Autodesk Inventor part; units mm, degrees
ref_plane "YZ Plane" through (0, 0, 0) normal (1, 0, 0) x (0, 1, 0)
ref_plane "XZ Plane" through (0, 0, 0) normal (0, 1, 0) x (-1, 0, 0)
ref_plane "XY Plane" through (0, 0, 0) normal (0, 0, 1) x (1, 0, 0)
sketch "Sketch1" plane through (0, 0, 0) normal (1, 0, 0) x (0, 1, 0)
  line L0 (0, 24.9554) -> (36.4449, 24.9554)
  arc A0 (31.5833, 1.489) -> (36.4449, 24.9554) centre (37.5, 12.5) ccw
  arc A1 (31.7956, 1.3803) -> (0, 9.582) centre (-2.2398, -64.8326) ccw
  circle A2 centre (37.5, 3.991) radius 1.25
  circle A3 centre (28.991, 12.5) radius 1.25
  circle A4 centre (37.5, 21.009) radius 1.25
  circle A5 centre (46.009, 12.5) radius 1.25
  circle A6 centre (28.6546, 17.1646) radius 1.25
  circle A7 centre (20.6937, 21.3627) radius 1.25
  circle A8 centre (37.5, 12.5) radius 4.5
  line L1 (-2.2398, 24.9554) -> (-2.25, 24.9554)
  arc A9 (-2.2398, 9.6157) -> (-2.25, 9.6157) centre (-2.2398, -64.8326) ccw
  arc A10 (0, 9.582) -> (-31.7956, 1.3803) centre (2.2398, -64.8326) ccw
  line L2 (0, 24.9554) -> (-36.4449, 24.9554)
  arc A11 (-36.4449, 24.9554) -> (-31.5833, 1.489) centre (-37.5, 12.5) ccw
  circle A12 centre (-37.5, 3.991) radius 1.25
  circle A13 centre (-28.991, 12.5) radius 1.25
  circle A14 centre (-37.5, 21.009) radius 1.25
  circle A15 centre (-46.009, 12.5) radius 1.25
  circle A16 centre (-28.6546, 17.1646) radius 1.25
  circle A17 centre (-20.6937, 21.3627) radius 1.25
  circle A18 centre (-37.5, 12.5) radius 4.5
  line L3 (2.2398, 24.9554) -> (2.25, 24.9554)
  arc A19 (2.25, 9.6157) -> (2.2398, 9.6157) centre (2.2398, -64.8326) ccw
  point P0 (0.0204, 0)
  point P1 (-0.0204, 0)
  dimension "d47" = 8.509
  dimension "d48" = 8.509
  dimension "d49" = 8.509
  dimension "d50" = 8.509
  dimension "d51" = 10
  dimension "d53" = 9
  dimension "d56" = 9
  dimension "d58" = 4.1981
  dimension "d61" = 75
extrude "Extrusion3" add sketch "Sketch1" along normal mid plane 3.5
properties part number "tibia extrude"
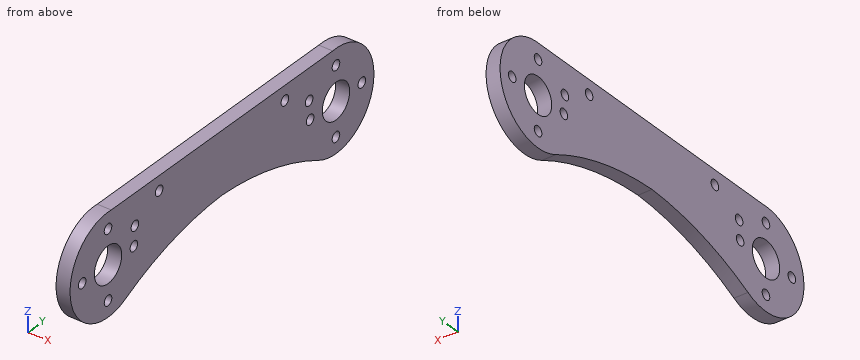
Work out the finished part from the listing and answer in its coordinate system (mm). Give positions to 0.01 mm unless a question says otherwise; leave off trailing zeros. Order: outer loops, then holes, each group sorted by start corner. A loop starts at its lowest first (then second) coordinate and runs counter-clockwise, first axis right, second up. Notation, with made-up numbers: (83.5, 87) -> (117.5, 87) arc R26 ccw to (117.5, 121) -> close; hole circle Ø6 at (55, 18). An arc over 180 degrees is marked (long way). One line per item, written item: value.
Item 1: Find section A-A, the plane z = 12.5. Give the vertices of the cut face in (x, y), plus the area to 3 significant figures.
Answer sheet:
outline: (-1.75, -50) -> (1.75, -50) -> (1.75, -47.26) -> (-1.75, -47.26) -> close; (-1.75, -44.76) -> (1.75, -44.76) -> (1.75, -42) -> (-1.75, -42) -> close; (-1.75, -33) -> (1.75, -33) -> (1.75, -30.24) -> (-1.75, -30.24) -> close; (-1.75, -27.74) -> (1.75, -27.74) -> (1.75, 27.74) -> (-1.75, 27.74) -> close; (-1.75, 30.24) -> (1.75, 30.24) -> (1.75, 33) -> (-1.75, 33) -> close; (-1.75, 42) -> (1.75, 42) -> (1.75, 44.76) -> (-1.75, 44.76) -> close; (-1.75, 47.26) -> (1.75, 47.26) -> (1.75, 50) -> (-1.75, 50) -> close
area: 252 mm²
Item 2: Flat-ended cylindrical pins translate along their axes: P1, Ø2, axis at y = 28.65, z = 17.16, coming from the -X side; P2, Ø1.5, axis at x = 1, z = 17.5, coming from the -Y side. Find the tip coordinate at first contact, or state that the pin passes through.
Answer sheet:
P1: through
P2: y = -49.26
Item 3: Find section C-C, the plane x = -0.6. State how many separate pieces and enclosed holes the cut face has, plus the area to 3 significant figures.
Answer sheet:
separate pieces: 1
enclosed holes: 14
area: 1,740 mm²
Item 4: Find section D-D, the plane y = 10. Give the vertices of the cut face in (x, z).
Answer sheet:
outline: (-1.75, 8.6) -> (1.75, 8.6) -> (1.75, 24.96) -> (-1.75, 24.96) -> close
Item 5: Straight lines are drawn through the part: probe 1 along Y at (x, z) = (1.5, 15.5); probe 2 along Y at (x, z) = (1.15, 15.75); probe 3 along Y at (x, z) = (1.05, 16.25). For each, find the intervals that lie inside material, in ascending order.
Answer sheet:
probe 1: -49.63 to -40.85, -34.15 to 34.15, 40.85 to 49.63
probe 2: -49.57 to -40.61, -34.39 to 34.39, 40.61 to 49.57
probe 3: -49.42 to -39.99, -35.01 to -29.51, -27.8 to 27.8, 29.51 to 35.01, 39.99 to 49.42
Item 6: Find section B-B, the plane y = -37.5. Give the vertices of the cut face in (x, z).
Answer sheet:
outline: (-1.75, 0) -> (1.75, 0) -> (1.75, 2.74) -> (-1.75, 2.74) -> close; (-1.75, 5.24) -> (1.75, 5.24) -> (1.75, 8) -> (-1.75, 8) -> close; (-1.75, 17) -> (1.75, 17) -> (1.75, 19.76) -> (-1.75, 19.76) -> close; (-1.75, 22.26) -> (1.75, 22.26) -> (1.75, 25) -> (-1.75, 25) -> close
